```python
from build123d import *

# Parameters (mm, degrees)
BOSS_EXTRUDE1_DEPTH         = 12.7
F_1_2_20_TAPPED_HOLE1_D     = 11.50874
F_1_2_20_TAPPED_HOLE1_DEPTH = 9.525


with BuildPart() as part:
    # Sketch2 → Boss-Extrude1 (new, symmetric)
    with BuildSketch(Plane.XY):
        with BuildLine():
            Line((0, -31.75), (50.8, -31.75))
            Line((50.8, -31.75), (50.8, 12.7))
            Line((50.8, 12.7), (19.05, 12.7))
            ThreePointArc((19.05, 12.7), (14.2875, 17.4625), (19.05, 22.225))
            Line((19.05, 22.225), (50.8, 22.225))
            Line((50.8, 22.225), (50.8, 31.75))
            Line((50.8, 31.75), (0, 31.75))
            Line((0, 31.75), (0, -12.7))
            Line((0, -12.7), (31.75, -12.7))
            ThreePointArc((31.75, -12.7), (36.5125, -17.4625), (31.75, -22.225))
            Line((31.75, -22.225), (0, -22.225))
            Line((0, -22.225), (0, -31.75))
        make_face()
    extrude(amount=BOSS_EXTRUDE1_DEPTH, both=True)

    # 1/2-20 Tapped Hole1
    with Locations(Plane(origin=(0, 31.75, 0), x_dir=(1, 0, 0), z_dir=(0, 1, 0))):
        with Locations((25.4, 0)):
            f_1_2_20_tapped_hole1 = Hole(F_1_2_20_TAPPED_HOLE1_D / 2, depth=F_1_2_20_TAPPED_HOLE1_DEPTH)

    # Mirror1: 1/2-20 Tapped Hole1 across plane
    add(f_1_2_20_tapped_hole1.mirror(Plane.ZX), mode=Mode.SUBTRACT)


solid = part.part
```
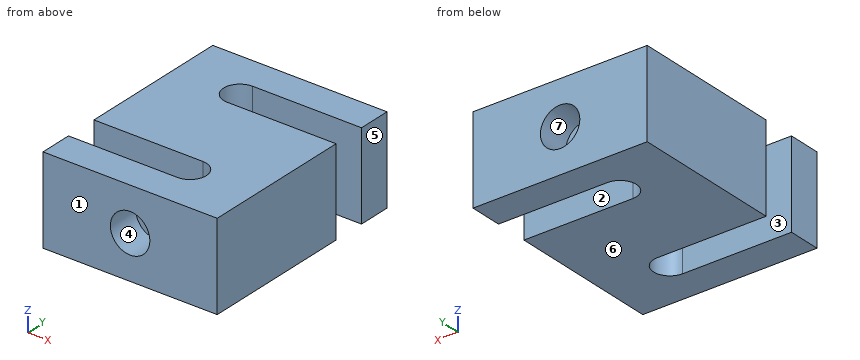
Geometry: final body of the model. Coordinates: model frame, mm. Face numbers are marked on the shaded views. A direction names the side the tool comes from. Round coordinates to 2 decimals unless told otherwise and drop trailing zeros. Order: outer loops, then holes, each group sorted by start corner. A loop starts at its lowest first (then second) coordinate and runs counter-clockwise, first axis right, second up. Notation, with made-up numbers: (84, -35) - (129, -35) arc R29 cw to (129, -2) - close; hole circle Ø7 at (-35, 72.25). An arc over 180 degrees is marked (long way). Write item = value, one per line. Start each with the question number.
Q1. Pin query (flat end, axial travel): pin 1 (9 mm diameter, centred on x = 25.4, z = 0, fed in from -Y). Return the tip coordinate at first contact, or that it passes through.
Q2. Pull-direction query (Z, two-part tool) for the marked faces 5, 6 and 7; classes: +Z half, -Z half, draft (parallel to the pull), parting line (faces both ways), or undercut.
Q3. Cut plane A-A on x = 39.5. Return the cut outline in (y, z) (3 decimals), and give its area (3 significant figures).
Q4. Cut plane D-D on y = 28.5. Return the cut outline in (x, z), and give its area (3 significant figures).
Q5. Ray query, line 1 (Y direction, x = 31.5, z = 8.5) (3 decimals); line 2 (Y direction, x = 33, z = 2.75) (3 decimals); line 3 (Z direction, x = 25.4, y = 26.5). Return the intervals inside material, ascending. Write a range as from..to.
Q6. Cut plane C-C on x = 25.4. Return the cut outline in (y, z) (3 decimals), and give its area (3 significant figures).
Q7. Access query for the marked faces 1, 2, 3 and 4. Directions: +Z, -Z, +X, -X, +Y, -Y. A direction counts if a zero-diameter tool reaches every point of the face in a straight line with its end or side. Return the directions, or none.
Q8. Cut plane B-B on z = 0. Give the number of separate pieces and of enclosed holes in the cut face, and give its area (3 significant figures).
Outcome:
q1.pin_1 = -12.7
q2.face_5 = draft
q2.face_6 = -Z half
q2.face_7 = undercut
q3.outline = (-31.75, -12.7) - (12.7, -12.7) - (12.7, 12.7) - (-31.75, 12.7) - close; (22.225, -12.7) - (31.75, -12.7) - (31.75, 12.7) - (22.225, 12.7) - close
q3.area = 1,370 mm^2
q4.outline = (0, -12.7) - (50.8, -12.7) - (50.8, 12.7) - (0, 12.7) - close; hole circle Ø11.51 at (25.4, 0)
q4.area = 1,190 mm^2
q5.line_1 = -31.75..-22.225, -12.7..12.7, 22.225..31.75
q5.line_2 = -31.75..-22.058, -12.867..12.7, 22.225..31.75
q5.line_3 = -12.7..-5.75, 5.75..12.7
q6.outline = (-31.75, -12.7) - (-22.225, -12.7) - (-22.225, -5.754) - (-31.75, -5.754) - close; (-31.75, 5.754) - (-22.225, 5.754) - (-22.225, 12.7) - (-31.75, 12.7) - close; (-12.7, -12.7) - (12.7, -12.7) - (12.7, 12.7) - (-12.7, 12.7) - close; (22.225, -12.7) - (31.75, -12.7) - (31.75, -5.754) - (22.225, -5.754) - close; (22.225, 5.754) - (31.75, 5.754) - (31.75, 12.7) - (22.225, 12.7) - close
q6.area = 910 mm^2
q7.face_1 = +Z, -Z, +X, -X, -Y
q7.face_2 = +Z, -Z, +X
q7.face_3 = +Z, -Z, -X
q7.face_4 = -Y
q8.separate_pieces = 3
q8.enclosed_holes = 0
q8.area = 2,330 mm^2
